```python
from build123d import *

# Parameters (mm, degrees)
SKETCH3_R          = 1.7
CUT_EXTRUDE1_DEPTH = 98.929821811
CIRPATTERN1_COUNT  = 3
CUT_EXTRUDE2_DEPTH = 3
CIRPATTERN2_COUNT  = 3


with BuildPart() as part:
    # Sketch2 → Revolve1 (revolve)
    with BuildSketch(Plane.XY):
        Polygon((53, 0), (68, 0), (68, 18.5), (55, 18.5), (55, 5.5), (49, 5.5), (49, 5), align=None)
    revolve(axis=Axis((0, -18.5, 0), (0, 1, 0)))

    # Sketch3 → Cut-Extrude1 (cut, through all)
    with BuildSketch(Plane(origin=(0, 18.5, 0), x_dir=(1, 0, 0), z_dir=(0, 1, 0))):
        with Locations(Location((0, 61.5, 0), (0, 0, 180))):
            Circle(SKETCH3_R)
    cut_extrude1 = extrude(amount=-CUT_EXTRUDE1_DEPTH, mode=Mode.SUBTRACT)

    # CirPattern1: Cut-Extrude1 ×3 about axis
    cirpattern1_axis = Axis((0, 0, 0), (0, 1, 0))
    for i in range(1, CIRPATTERN1_COUNT):
        add(cut_extrude1.rotate(cirpattern1_axis, i * 360 / CIRPATTERN1_COUNT), mode=Mode.SUBTRACT)

    # Sketch4 → Cut-Extrude2 (cut)
    with BuildSketch(Plane.XZ):
        Polygon((-54.935562333, 33.651185103), (-56.610562333, 30.75), (-54.935562333, 27.848814897), (-51.585562333, 27.848814897), (-49.910562333, 30.75), (-51.585562333, 33.651185103), align=None)
    cut_extrude2 = extrude(amount=-CUT_EXTRUDE2_DEPTH, mode=Mode.SUBTRACT)

    # CirPattern2: Cut-Extrude2 ×3 about axis
    cirpattern2_axis = Axis((0, 0, 0), (0, 1, 0))
    for i in range(1, CIRPATTERN2_COUNT):
        add(cut_extrude2.rotate(cirpattern2_axis, i * 360 / CIRPATTERN2_COUNT), mode=Mode.SUBTRACT)


solid = part.part
```
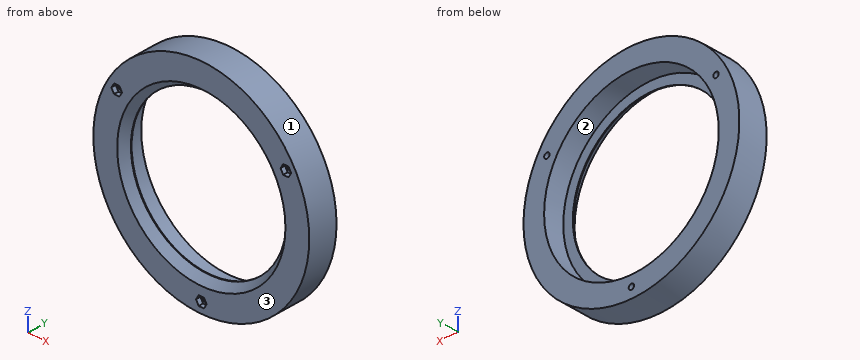
Input: part model. Units: mm. Frame: model coordinates. Face numbers are marked on the shaded views. Give positions to 0.01 mm unless a question says otherwise; leave off trailing zeros. Order: outer loops, then holes, each group sorted by start corner. A loop starts at its lowest first (then second) coordinate and runs counter-clockwise, first axis right, second up. Notation, with made-up numbers: M 50.5,16.5 L 66.5,16.5 A13 ccw 66.5,41.5 Z; hole C 71,17.25 d8. An arc over 180 degrees is marked long. Return JSON: item names as keys, results as strings.
Item 1: Pull-direction query (Z, two-part tool) for the marked faces 1, 2 and 3; classes: +Z half, -Z half, draft (parallel to the pull), parting line (faces both ways), or undercut.
Solutions:
{"face 1": "parting line", "face 2": "undercut", "face 3": "draft"}
Item 2: Cut plane B-B (z = 0). Return loops of the section in (x, y), then the cut area to 3 significant figures.
Solutions:
{"outline": "M -68,0 L -53,0 L -49,5 L -49,5.5 L -55,5.5 L -55,18.5 L -68,18.5 Z; M 49,5 L 53,0 L 68,0 L 68,18.5 L 55,18.5 L 55,5.5 L 49,5.5 Z", "area": "527 mm^2"}
Item 3: Cut plane A-A (x = 0). Return loops of the section in (y, z), then the cut area to 3 significant figures.
Solutions:
{"outline": "M 0,-68 L 18.5,-68 L 18.5,-63.2 L 3,-63.2 L 3,-64.4 L 0,-64.4 Z; M 0,-58.6 L 3,-58.6 L 3,-59.8 L 18.5,-59.8 L 18.5,-55 L 5.5,-55 L 5.5,-49 L 5,-49 L 0,-53 Z; M 0,53 L 5,49 L 5.5,49 L 5.5,55 L 18.5,55 L 18.5,68 L 0,68 Z", "area": "457 mm^2"}
Item 4: Ray query, probe 1 along Z at (x, y) = (0, 5.2); probe 2 along Z at (x, y) = (0, 11.25); probe 3 along X at (y, z) = (12.25, 0). Return the intervals inside material, ascending.
Solutions:
{"probe 1": "-68 to -63.2, -59.8 to -49, 49 to 68", "probe 2": "-68 to -63.2, -59.8 to -55, 55 to 68", "probe 3": "-68 to -55, 55 to 68"}
Item 5: First-contact query: P1, Ø0.9, axis at x = 0.5, y = 1.5, coming from the -Z side; P2, Ø1.7, axis at x = 1.5, z = -61, coming from the -Y side; P3, Ø1.5, axis at x = 53.5, y = 1.5, coming from the +Z side; P4, Ø4, axis at x = -53.26, z = 30.75, coming from the +Y side. Flat tips, straight axial feed; report the tip coordinate or a pass-through.
Solutions:
{"P1": "z = -68", "P2": "y = 3", "P3": "z = 42.91", "P4": "y = 18.5"}
Item 6: Cut plane C-C (y = 7.5). Return loops of the section in (x, z).
Solutions:
{"outline": "C 0,0 d136; hole C 0,0 d110; hole C -53.26,30.75 d3.4; hole C 0,-61.5 d3.4; hole C 53.26,30.75 d3.4"}
